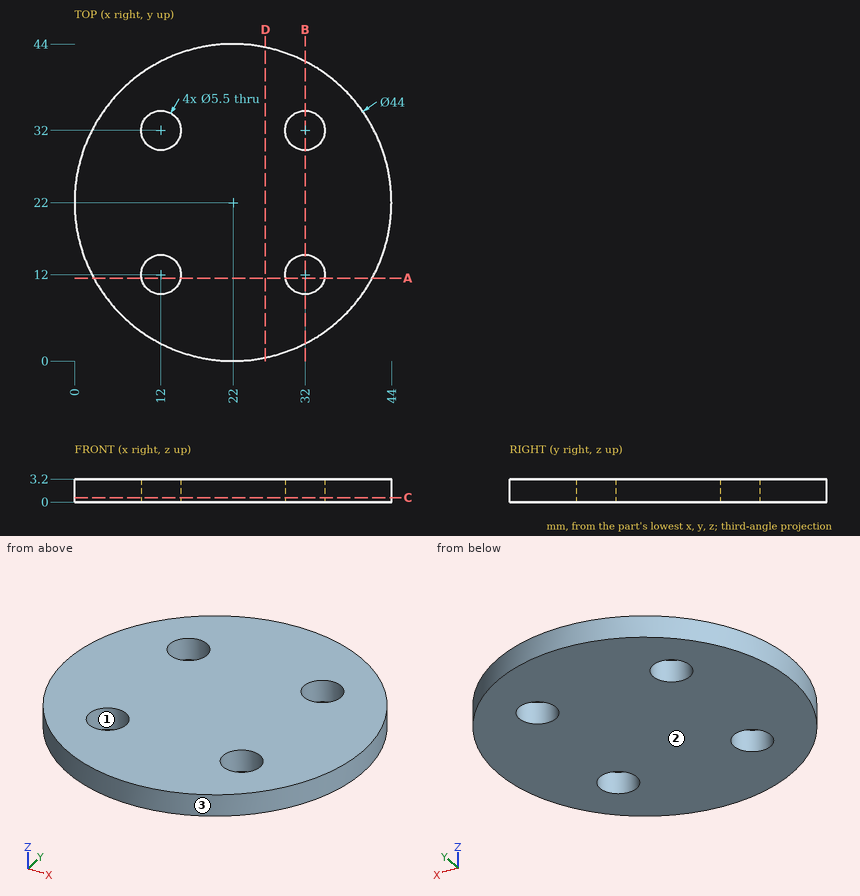
Can you work these out from the drawing? Everything is in mm from the part's minimum corner. Give positions to 0.01 mm unless a question says otherwise; leave off trailing zeros. Order: outer loops, then holes, each group sorted by start corner. A loop starts at its lowest first (then second) coordinate and runs counter-clockwise, first axis right, second up.
1. Will these pins go through, and if not, where does the flat tip stop? P1, Ø6, axis at x = 16.5, y = 8, coming from the -Z side; P2, Ø1.5, axis at x = 10.5, z = 2, coming from the -Y side.
2. Suppose I cut it at D-D (x = 26.5). List the corners of the cut face in (y, z) for me.
3. Suppose I cut it at C-C (z = 0.6). List the corners of the cut face in (x, y) for me.
4. Suppose I cut it at B-B (x = 32). List the corners of the cut face in (y, z) for me.
5. We'd pull the mould along Y, two halves only. Please class the marked faces 1, 2 and 3: pulls with the +Y half, pulls with the -Y half, needs draft (parallel to the pull), parting line crosses it, or undercut.
6. I need wall thicknesses on L1, parallel to X at y = 32, z = 1.8; L2, parallel to Y at x = 31, z = 2.9; L3, parallel to X at y = 10.5, z = 0.2 (3 decimals). Which ranges of each line are inside material? Lowest first, please.
7. Suppose I cut it at A-A (y = 11.5). List the corners of the cut face in (x, z) for me.
Solved:
1. P1: stops at z = 0
1. P2: stops at y = 2.81
2. outline: (0.47, 0) - (43.53, 0) - (43.53, 3.2) - (0.47, 3.2) - close
3. outline: circle Ø44 at (22, 22); hole circle Ø5.5 at (12, 12); hole circle Ø5.5 at (12, 32); hole circle Ø5.5 at (32, 12); hole circle Ø5.5 at (32, 32)
4. outline: (2.4, 0) - (9.25, 0) - (9.25, 3.2) - (2.4, 3.2) - close; (14.75, 0) - (29.25, 0) - (29.25, 3.2) - (14.75, 3.2) - close; (34.75, 0) - (41.6, 0) - (41.6, 3.2) - (34.75, 3.2) - close
5. face 1: undercut
5. face 2: needs draft
5. face 3: parting line crosses it
6. L1: x = 2.4 to 9.25, 14.75 to 29.25, 34.75 to 41.6
6. L2: y = 1.93 to 9.44, 14.56 to 29.44, 34.56 to 42.07
6. L3: x = 3.245 to 9.695, 14.305 to 29.695, 34.305 to 40.755
7. outline: (2.67, 0) - (9.3, 0) - (9.3, 3.2) - (2.67, 3.2) - close; (14.7, 0) - (29.3, 0) - (29.3, 3.2) - (14.7, 3.2) - close; (34.7, 0) - (41.33, 0) - (41.33, 3.2) - (34.7, 3.2) - close
